Geometry: final body of the model. Coordinates: model frame, mm. Face numbers are marked on the shaded views. A direction names the side the tool comes from. Coordinates: 2 decimals unless noted, no trailing zeros. Order: outer loops, then holes, each group sorted by start corner. A loop starts at its lowest first (then second) coordinate and runs counter-clockwise, first axis right, second up. Notation, with made-up numbers: (-11, 39.5) -> (42, 39.5) arc R27 ccw to (42, 68.5) -> close; hole circle Ø8 at (-15.75, 38). An arc over 180 degrees is marked (long way). Use one line per item in the form item = value.
Autodesk Inventor part; units mm, degrees
ref_plane "Work Plane1" through (0, 0, 16) normal (0, 0, 1) x (1, 0, 0)
ref_plane "YZ Plane" through (0, 0, 0) normal (1, 0, 0) x (0, 1, 0)
ref_plane "XZ Plane" through (0, 0, 0) normal (0, 1, 0) x (-1, 0, 0)
sketch "Sketch1" plane through (0, 0, 0) normal (0, 0, 1) x (1, 0, 0)
  line L0 (-36.8533, 0) -> (46.8153, 0) construction
  line L1 (0, -29.8808) -> (0, 4.9801) construction
  line L2 (0, 0) -> (24.6516, -24.6516) construction
  line L3 (0, 0) -> (34.8626, 0) construction
  line L4 (0, -24.9006) -> (16.8, -24.9006)
  line L5 (16.8, -24.9006) -> (16.8, -21.2406)
  line L6 (16.8, -21.2406) -> (19.0203, -19.0203)
  line L7 (24.9006, 0) -> (24.9006, -16.8)
  line L8 (24.9006, -16.8) -> (21.2406, -16.8)
  line L9 (21.2406, -16.8) -> (19.0203, -19.0203)
  line L10 (0, 0) -> (-24.6516, -24.6516) construction
  line L11 (0, -24.9006) -> (-16.8, -24.9006)
  line L12 (-16.8, -24.9006) -> (-16.8, -21.2406)
  line L13 (-16.8, -21.2406) -> (-19.0203, -19.0203)
  line L14 (-24.9006, 0) -> (-24.9006, -16.8)
  line L15 (-24.9006, -16.8) -> (-21.2406, -16.8)
  line L16 (-21.2406, -16.8) -> (-19.0203, -19.0203)
  arc A0 (-14, 0) -> (14, 0) centre (0, 0) ccw
  line L17 (0, 0) -> (14, 0) construction
  line L18 (0, 0) -> (-14, 0) construction
  line L19 (-14, 0) -> (-24.9006, 0)
  line L20 (14, 0) -> (24.9006, 0)
  dimension "d0" = 45
  dimension "d1" = 16.8
  dimension "d2" = 3.66
  dimension "d4" = 3.14
  dimension "d5" = 14
  dimension "d6" = 180
extrude "Extrusion1" add sketch "Sketch1" along normal blind 5
sketch "Sketch3" plane through (-24.9006, 0, 0) normal (0, 1, 0) x (1, 0, 0)
  line L0 (10.9006, 0) -> (0, 0) construction
  line L1 (0, 0) -> (0, -5) construction
  line L2 (10.9006, -5) -> (0, -5) construction
  line L3 (10.9006, 0) -> (10.9006, -5) construction
  line L4 (38.9006, 0) -> (10.9006, 0) construction
  line L5 (10.9006, 0) -> (10.9006, -5) construction
  line L6 (38.9006, -5) -> (10.9006, -5) construction
  line L7 (38.9006, 0) -> (38.9006, -5) construction
  line L8 (49.8013, 0) -> (38.9006, 0) construction
  line L9 (38.9006, 0) -> (38.9006, -5) construction
  line L10 (49.8013, -5) -> (38.9006, -5) construction
  line L11 (49.8013, 0) -> (49.8013, -5) construction
  line L12 (24.9006, 18.5006) -> (24.9006, -23.5037) construction
  arc A0 (10.9006, 0) -> (24.9006, -14) centre (24.9006, 0) ccw
  arc A1 (8.9006, 0) -> (24.9006, -16) centre (24.9006, 0) ccw
  line L13 (24.9006, -16) -> (24.9006, -14)
  line L14 (10.9006, 0) -> (0, 0)
  line L15 (8.9006, 0) -> (10.9006, 0)
  dimension "d11" = 2
revolve "Revolution2" add sketch "Sketch3" angle 180 about axis through (0, 0, -10) along (0, 0, 1)
ref_plane "Work Plane1" through (0, 0, 16) normal (0, 0, 1) x (1, 0, 0)
sketch "Sketch5" plane through (24.9006, 0, 5) normal (0, 1, 0) x (1, 0, 0)
  line L0 (0, 0) -> (-9.7019, 0) construction
  line L1 (0, 5) -> (0, 0) construction
  line L2 (0, 5) -> (-10.9006, 5) construction
  arc A0 (-38.9006, 5) -> (-10.9006, 5) centre (-24.9006, 5) ccw construction
  line L3 (-38.9006, 5) -> (-49.8013, 5) construction
  line L4 (-49.8013, 5) -> (-49.8013, 0) construction
  line L5 (-40.0993, 0) -> (-49.8013, 0) construction
  arc A1 (-40.0993, 0) -> (-9.7019, 0) centre (-24.9006, 5) ccw construction
  arc A2 (-38.9006, 5) -> (-10.9006, 5) centre (-24.9006, 5) ccw construction
  line L6 (-10.9006, 5) -> (-38.9006, 5) construction
  line L7 (-24.9006, 25) -> (-24.9006, -17) construction
  line L8 (-24.9006, -6) -> (-35.7006, -6)
  line L9 (-35.7006, -6) -> (-35.7006, -8.1)
  line L10 (-35.7006, -8.1) -> (-24.9006, -8.1)
  line L11 (-24.9006, -8.1) -> (-24.9006, -6)
  arc A3 (-10.9006, 5) -> (-38.9006, 5) centre (-24.9006, 5) ccw construction
  line L12 (-24.9006, 19) -> (-24.9006, -6) construction
  line L13 (-24.9006, 19) -> (0.0994, 19) construction
  line L14 (-34.7006, -6) -> (-33.5609, -6)
  line L15 (-33.5609, -6) -> (-33.5609, -4.998)
  line L16 (-33.5609, -4.998) -> (-34.7006, -4.998)
  line L17 (-34.7006, -4.998) -> (-34.7006, -6)
  arc A4 (-38.9006, 5) -> (-10.9006, 5) centre (-24.9006, 5) ccw
  line L18 (-24.9006, -8.1) -> (-34.087, -8.1)
  line L19 (-34.087, -8.1) -> (-34.087, -11)
  line L20 (-34.087, -11) -> (-24.9006, -11)
  line L21 (-24.9006, -11) -> (-24.9006, -8.1)
  arc A5 (-40.0993, 0) -> (-9.7019, 0) centre (-24.9006, 5) ccw
  dimension "d16" = 10.8
  dimension "d17" = 2.1
  dimension "d19" = 25
  dimension "d20" = 90
  dimension "d21" = 1
revolve "Revolution3" cut sketch "Sketch5" angle 360 about axis through (0, 0, -10) along (0, 0, 1) contours L11 L10 A4 L8 | A4 L10 A5 L9 L8 | L8 L17 A4 | L21 A4 L10 | A4 L21 A5 L10 | L10 L9 A5
sketch "Sketch6" plane through (-24.9006, 0, 5) normal (0, 1, 0) x (1, 0, 0)
  line L0 (14.1006, -6.8051) -> (14.1006, -6) construction
  line L1 (14.1006, -6) -> (15.1006, -6) construction
  line L2 (15.1006, -6) -> (15.1006, -4.998) construction
  arc A0 (10.9006, 5) -> (15.1006, -4.998) centre (24.9006, 5) ccw construction
  line L3 (10.9006, 5) -> (0, 5) construction
  line L4 (0, 5) -> (0, 0) construction
  line L5 (9.7019, 0) -> (0, 0) construction
  arc A1 (9.7019, 0) -> (14.1006, -6.8051) centre (24.9006, 5) ccw construction
  line L6 (24.9006, 7.4176) -> (24.9006, -9.5058) construction
  arc A2 (9.7019, 0) -> (14.1006, -6.8051) centre (24.9006, 5) ccw
  line L7 (13.2817, -6) -> (13.2817, -9.314)
  line L8 (14.1006, -6) -> (24.9006, -6) construction
  line L9 (24.9006, -6) -> (24.9006, -8) construction
  line L10 (24.9006, -8) -> (14.1006, -8) construction
  line L11 (14.1006, -8) -> (14.1006, -6) construction
  line L12 (35.7006, -6) -> (14.1006, -6) construction
  line L13 (14.1006, -6) -> (24.9006, -6) construction
  line L14 (24.9006, -6) -> (24.9006, -11.2) construction
  line L15 (24.9006, -11.2) -> (14.1006, -11.2) construction
  line L16 (14.1006, -11.2) -> (14.1006, -6) construction
  arc A3 (14.1006, -8) -> (24.9006, -11.2) centre (24.9006, 8.625) ccw construction
  line L17 (14.1006, -6.8051) -> (14.1006, -8)
  line L18 (13.2817, -9.314) -> (15.1006, -9.314)
  line L19 (15.1006, -9.314) -> (15.1006, -8.6084)
  line L20 (15.1006, -8.6084) -> (14.1006, -8)
  line L21 (13.2817, -6) -> (14.1006, -6)
  line L22 (35.7006, -6.8051) -> (14.1006, -6.8051)
  line L23 (14.1006, -6.8051) -> (14.1006, -6)
  dimension "d23" = 2
  dimension "d24" = 5.2
revolve "Revolution4" add sketch "Sketch6" angle 180 about axis through (0, 0, -10) along (0, 0, 1) contours A2 L17 L20 L19 L18 L7
sketch "Sketch7" plane through (0, 0, 0) normal (0, 0, -1) x (-1, 0, 0)
  line L0 (-24.9006, 0) -> (-14, 0)
  line L1 (-24.9006, -16.8) -> (-24.9006, 0)
  line L2 (-21.2406, -16.8) -> (-24.9006, -16.8)
  line L3 (-16.8, -21.2406) -> (-21.2406, -16.8)
  line L4 (-16.8, -24.9006) -> (-16.8, -21.2406)
  line L5 (16.8, -24.9006) -> (-16.8, -24.9006)
  line L6 (16.8, -21.2406) -> (16.8, -24.9006)
  line L7 (21.2406, -16.8) -> (16.8, -21.2406)
  line L8 (24.9006, -16.8) -> (21.2406, -16.8)
  line L9 (24.9006, 0) -> (24.9006, -16.8)
  line L10 (14, 0) -> (24.9006, 0)
  arc A0 (-14, 0) -> (14, 0) centre (0, 0) ccw
extrude "Extrusion3" add sketch "Sketch7" along normal blind 7
properties part number "20_Cube_Insert_Eye_Lens"
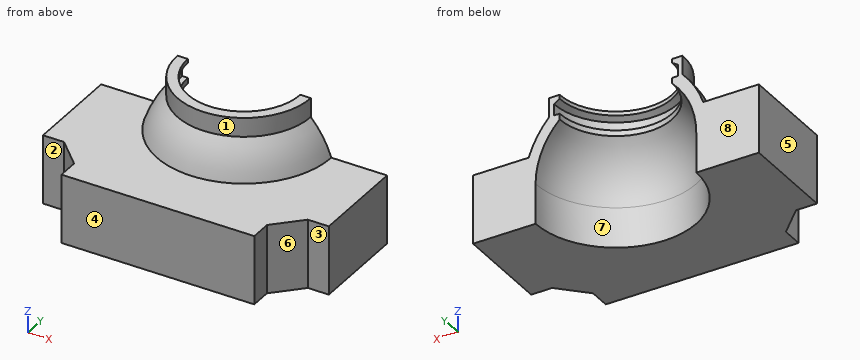
1) Access query for the marked faces 1, 2, 3 and 4. Directions: +Z, -Z, +X, -X, +Y, -Y. A direction counts if a zero-diameter tool reaches every point of the face in a straight line with its end or side. Return the directions, or none.
Results found:
face_1 = +Z, -Y
face_2 = +Z, -Z, -X, -Y
face_3 = +Z, -Z, +X, -Y
face_4 = +Z, -Z, +X, -X, -Y
2) Pull-direction query (X, two-part tool) for the marked faces 5, 6, 7 and 8; classes: released by +X, released by -X, zero draft, split by the parting line, or undercut.
Results found:
face_5 = released by -X
face_6 = released by +X
face_7 = undercut
face_8 = zero draft
3) Section C-C, the plane x = 0. Output: boundary loops of the cut face in (y, z).
Results found:
outline = (-24.9, -7) -> (-14, -7) -> (-14, 0) arc R14 cw to (-9.8, 10) -> (-9.8, 11) -> (-10.8, 11) -> (-10.8, 13) -> (-9.8, 13.61) -> (-9.8, 14.31) -> (-11.62, 14.31) -> (-11.62, 11) arc R16 ccw to (-15.2, 5) -> (-24.9, 5) -> close
4) Material intervals for probe 1 along X at (y, z) = (-8.25, 9.75); probe 2 along Z at (x, y) = (16, -20.75); probe 3 along X at (y, z) = (-2.75, 7), sorted ascending. Write a range as from..to.
Results found:
probe_1 = -9.64..-5.73, 5.73..9.64
probe_2 = -7..5
probe_3 = -14.12..-11.81, 11.81..14.12
5) Section B-B, the plane y = -23. Output: boundary loops of the cut face in (x, z).
Results found:
outline = (-16.8, -7) -> (16.8, -7) -> (16.8, 5) -> (-16.8, 5) -> close
6) Contact query for flat-ended pins moving along their axis: P1, Ø4, axis at x = -22.5, z = -3, coming from the -Y side; P2, Ø4, axis at y = -10.5, z = 9, coming from the +X side; P3, Ø4, axis at y = -23.5, z = -2.5, coming from the +X side. Output: stop coordinate, or through.
Results found:
P1 = -17.54
P2 = 10.77
P3 = 16.8
7) Section D-D, the plane z = 12. Output: boundary loops of the cut face in (x, y).
Results found:
outline = (-11.62, 0) arc R11.62 ccw to (11.62, 0) -> (10.8, 0) arc R10.8 cw to (-10.8, 0) -> close
8) Section A-A, the plane z = -3.25. Output: boundary loops of the cut face in (x, y).
Results found:
outline = (-24.9, -16.8) -> (-21.24, -16.8) -> (-16.8, -21.24) -> (-16.8, -24.9) -> (16.8, -24.9) -> (16.8, -21.24) -> (21.24, -16.8) -> (24.9, -16.8) -> (24.9, 0) -> (14, 0) arc R14 cw to (-14, 0) -> (-24.9, 0) -> close
